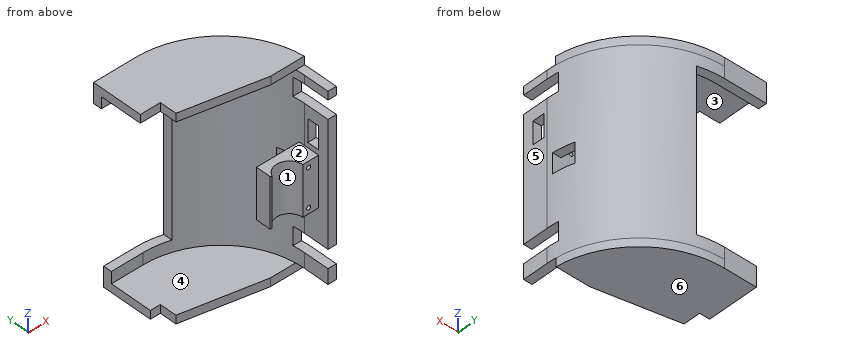
```python
from build123d import *

# Parameters (mm, degrees)
BOSS_EXTRUDE1_DEPTH     = 110
SKETCH2_W               = 30
SKETCH2_H               = 12.5
BOSS_EXTRUDE2_DEPTH     = 35
SKETCH3_R               = 8
CUT_EXTRUDE1_DEPTH      = 121.603742452
SKETCH4_R               = 1.5
SKETCH4_R_2             = 1.25
CUT_EXTRUDE2_DEPTH      = 12.5
SKETCH5_W               = 9.5
SKETCH5_H               = 12.5
CUT_EXTRUDE3_DEPTH      = 121.603742452
FILLET4_R               = 0.5
BOSS_EXTRUDE3_DEPTH     = 5
CUT_EXTRUDE4_DEPTH      = 158.919156753
CUT_EXTRUDE4_DEPTH_BACK = 158.919156753
SKETCH7_W               = 12
SKETCH7_H               = 12
SKETCH7_W_2             = 11
SKETCH7_H_2             = 22
SKETCH7_W_3             = 13.6
SKETCH7_H_3             = 7
BOSS_EXTRUDE4_START     = 5
BOSS_EXTRUDE4_DEPTH     = 5
CUT_EXTRUDE5_DEPTH      = 152.478720037


with BuildPart() as part:
    # Sketch1 → Boss-Extrude1 (new body)
    with BuildSketch(Plane.XY):
        with BuildLine():
            Line((13.568, -0.541666667), (18.568, -0.541666667))
            Line((18.568, -0.541666667), (18.568, 14.458333333))
            ThreePointArc((18.568, 14.458333333), (2.458872965, 53.349206299), (-36.432, 69.458333333))
            Line((-36.432, 69.458333333), (-69.432, 69.458333333))
            Line((-69.432, 69.458333333), (-69.432, 64.458333333))
            Line((-69.432, 64.458333333), (-36.432, 64.458333333))
            ThreePointArc((-36.432, 64.458333333), (-1.076660941, 49.813672393), (13.568, 14.458333333))
            Line((13.568, 14.458333333), (13.568, -0.541666667))
        make_face()
    extrude(amount=BOSS_EXTRUDE1_DEPTH)

    # Sketch2 → Boss-Extrude2 (add)
    with BuildSketch(Plane.ZY.offset(-13.568)):
        with Locations((55, 11.708333333)):
            Rectangle(SKETCH2_W, SKETCH2_H)
    extrude(amount=BOSS_EXTRUDE2_DEPTH)

    # Sketch3 → Cut-Extrude1 (cut, through all)
    with BuildSketch(Plane(origin=(0, 0, 40), x_dir=(-1, 0, 0), z_dir=(0, 0, -1))):
        with Locations((3.932, 5.458333333)):
            Circle(SKETCH3_R)
    extrude(amount=-CUT_EXTRUDE1_DEPTH, mode=Mode.SUBTRACT)

    # Sketch4 → Cut-Extrude2 (cut)
    with BuildSketch(Plane.XZ.offset(-5.458333333)):
        with Locations(Location((-17.932, 43.5, 0), (0, 0, 270))):
            Circle(SKETCH4_R)
        with Locations(Location((-17.932, 66.5, 0), (0, 0, 270))):
            Circle(SKETCH4_R)
        with Locations(Location((7.568, 43.5, 0), (0, 0, 270))):
            Circle(SKETCH4_R_2)
        with Locations(Location((7.568, 66.5, 0), (0, 0, 270))):
            Circle(SKETCH4_R_2)
    extrude(amount=-CUT_EXTRUDE2_DEPTH, mode=Mode.SUBTRACT)

    # Sketch5 → Cut-Extrude3 (cut, through all)
    with BuildSketch(Plane(origin=(0, 0, 40), x_dir=(-1, 0, 0), z_dir=(0, 0, -1))):
        with Locations((16.682, 11.708333333)):
            Rectangle(SKETCH5_W, SKETCH5_H)
    extrude(amount=-CUT_EXTRUDE3_DEPTH, mode=Mode.SUBTRACT)

    # Fillet4
    fillet4_edges = [part.edges().sort_by_distance(p)[0] for p in [
        (-11.932, 5.458333333, 55),
    ]]
    fillet(fillet4_edges, radius=FILLET4_R)

    # Sketch6 → Boss-Extrude3 (add)
    with BuildSketch(Plane.XY.offset(110)):
        with BuildLine():
            Line((18.310426703, 19.774978769), (-1.689573297, 19.774978769))
            Line((-1.689573297, 19.774978769), (-49.432, 29.458333333))
            Line((-49.432, 29.458333333), (-49.432, 39.458333333))
            Line((-49.432, 39.458333333), (-69.432, 39.458333333))
            Line((-69.432, 39.458333333), (-69.432, 69.458333333))
            Line((-69.432, 69.458333333), (-36.432, 69.458333333))
            ThreePointArc((-36.432, 69.458333333), (0.531390679, 55.1855693), (18.310426703, 19.774978769))
        make_face()
    extrude(amount=BOSS_EXTRUDE3_DEPTH)

    # Sketch7 → Cut-Extrude4 (cut, two sides: drawn at the far end of the back side and taken through both)
    with BuildSketch(Plane.ZY.offset(-13.568).offset(-CUT_EXTRUDE4_DEPTH_BACK)):
        with Locations((55, 23.958333333)):
            Rectangle(SKETCH7_W, SKETCH7_H)
        with Locations((99.5, 10.458333333)):
            Rectangle(SKETCH7_W_2, SKETCH7_H_2)
        with Locations((14.5, 10.458333333)):
            Rectangle(SKETCH7_W_2, SKETCH7_H_2)
        with Locations((79.8, 8.958333333)):
            Rectangle(SKETCH7_W_3, SKETCH7_H_3)
    extrude(amount=CUT_EXTRUDE4_DEPTH + CUT_EXTRUDE4_DEPTH_BACK, mode=Mode.SUBTRACT)

    # Sketch8 → Boss-Extrude4 (add)
    with BuildSketch(Plane(origin=(0, 0, 0), x_dir=(-1, 0, 0), z_dir=(0, 0, -1)).offset(BOSS_EXTRUDE4_START)):
        with BuildLine():
            Line((36.432, 69.458333333), (69.432, 69.458333333))
            Line((69.432, 69.458333333), (69.432, 64.458333333))
            Line((69.432, 64.458333333), (69.432, 39.458333333))
            Line((69.432, 39.458333333), (49.432, 39.458333333))
            Line((49.432, 39.458333333), (49.432, 29.458333333))
            Line((49.432, 29.458333333), (1.707690959, 19.958333333))
            Line((1.707690959, 19.958333333), (-18.292309041, 19.958333333))
            ThreePointArc((-18.292309041, 19.958333333), (-0.463121629, 55.247425012), (36.432, 69.458333333))
        make_face()
    extrude(amount=-BOSS_EXTRUDE4_DEPTH)

    # Sketch9 → Cut-Extrude5 (cut, through all)
    with BuildSketch(Plane(origin=(0, 69.458333333, 0), x_dir=(1, 0, 0), z_dir=(0, 1, 0))):
        Polygon((-55.432, -7), (-21.432, -7), (-21.432, -103), (-61.432, -103), (-61.432, -133.715891386), (-92.425116466, -133.715891386), (-92.425116466, -103), (-92.425116466, -7), (-92.425116466, 8.214128056), (-55.432, 8.214128056), align=None)
    extrude(amount=-CUT_EXTRUDE5_DEPTH, mode=Mode.SUBTRACT)


solid = part.part
```
Read the model definition and answer for the solid it produces. Units are mm, in the model's axes. Face numbers are marked on the shaded views. A direction names the side the tool comes from. Coordinates: 2 decimals unless noted, no trailing zeros. Loops run counter-clockwise (first coordinate to the right, second up) from the corner with the lowest first, then second, coordinate; pieces in that order, holes last. Notation, with made-up numbers: (24.5, 41) -> (28.5, 41) arc R16 ccw to (28.5, 52) -> close; hole circle Ø8 at (89, 87.5). An arc over 180 degrees is marked (long way). Return JSON: item names as keys, results as strings.
Item 1: Find section A-A (y = 26). Determine the outline of the cut face in (x, z).
Answers:
{"outline": "(-32.38, 110) -> (12.22, 110) -> (12.22, 61) -> (17.34, 61) -> (17.34, 115) -> (-32.38, 115) -> close; (-32.06, -5) -> (17.34, -5) -> (17.34, 49) -> (12.22, 49) -> (12.22, 0) -> (-32.06, 0) -> close"}
Item 2: Find section C-C (x = -34). Determine the outline of the cut face in (y, z).
Answers:
{"outline": "(26.33, 110) -> (64.4, 110) -> (64.4, 103) -> (69.4, 103) -> (69.4, 115) -> (26.33, 115) -> close; (26.39, -5) -> (69.4, -5) -> (69.4, 7) -> (64.4, 7) -> (64.4, 0) -> (26.39, 0) -> close"}
Item 3: Find the intervals of material crossed by probe 1 along Z at (x, y) = (-47.5, 32.5); probe 2 along X at (y, z) = (12, 66); probe 3 along Z at (x, y) = (-11, 12), in increasing order.
Answers:
{"probe 1": "z = -5 to 0, 110 to 115", "probe 2": "x = -11.93 to -8.54, 0.67 to 6.42, 8.71 to 18.57", "probe 3": "z = 40 to 70"}
Item 4: For the marked faces 1, 2 and 3, determine the directions among +Z, -Z, +X, -X, +Y, -Y from which every point of the face is accessible in a straight line to the end or side of a thin tool.
Answers:
{"face 1": "+Z, -Z, -Y", "face 2": "+Z, -X, -Y", "face 3": "-X, -Y"}
Item 5: For a pull along Z with two mould halves and no side action, classify the marked faces 4, 5 and 6 as +Z half, -Z half, draft (parallel to the pull), parting line (faces both ways), or undercut.
Answers:
{"face 4": "undercut", "face 5": "draft", "face 6": "-Z half"}
Item 6: Flat-ended cylindrical pins translate along their axes: P1, Ø1.5, axis at x = 16.5, z = 16.5, coming from the -Y side; P2, Ø14, axis at x = -0.5, y = 11.5, coming from the -Z side; P3, Ø1, axis at y = 30.5, z = 31.5, coming from the -X side. Find the tip coordinate at first contact, or state that the pin passes through.
Answers:
{"P1": "stops at y = 21.46", "P2": "stops at z = 40", "P3": "stops at x = 10.75"}
Item 7: Find section D-D (y = 51.5). Determine the outline of the cut face in (x, z).
Answers:
{"outline": "(-61.43, 110) -> (-2.85, 110) -> (-2.85, 0) -> (-55.43, 0) -> (-55.43, -5) -> (4.22, -5) -> (4.22, 115) -> (-61.43, 115) -> close"}
Item 8: Find section B-B (z = 53). Determine the outline of the cut face in (x, y), plus the area to 3 significant figures.
Answers:
{"outline": "(-21.43, 62.16) arc R50 cw to (11.1, 29.96) -> (16.34, 29.96) arc R55 ccw to (-21.43, 67.37) -> close; (-11.93, 9.46) arc R0.5 ccw to (-10.99, 9.22) arc R8 cw to (4.07, 5.46) -> (13.57, 5.46) -> (13.57, -0.54) -> (18.57, -0.54) -> (18.57, 14.46) arc R55 ccw to (18.46, 17.96) -> (-11.93, 17.96) -> close", "area": "567 mm2"}
